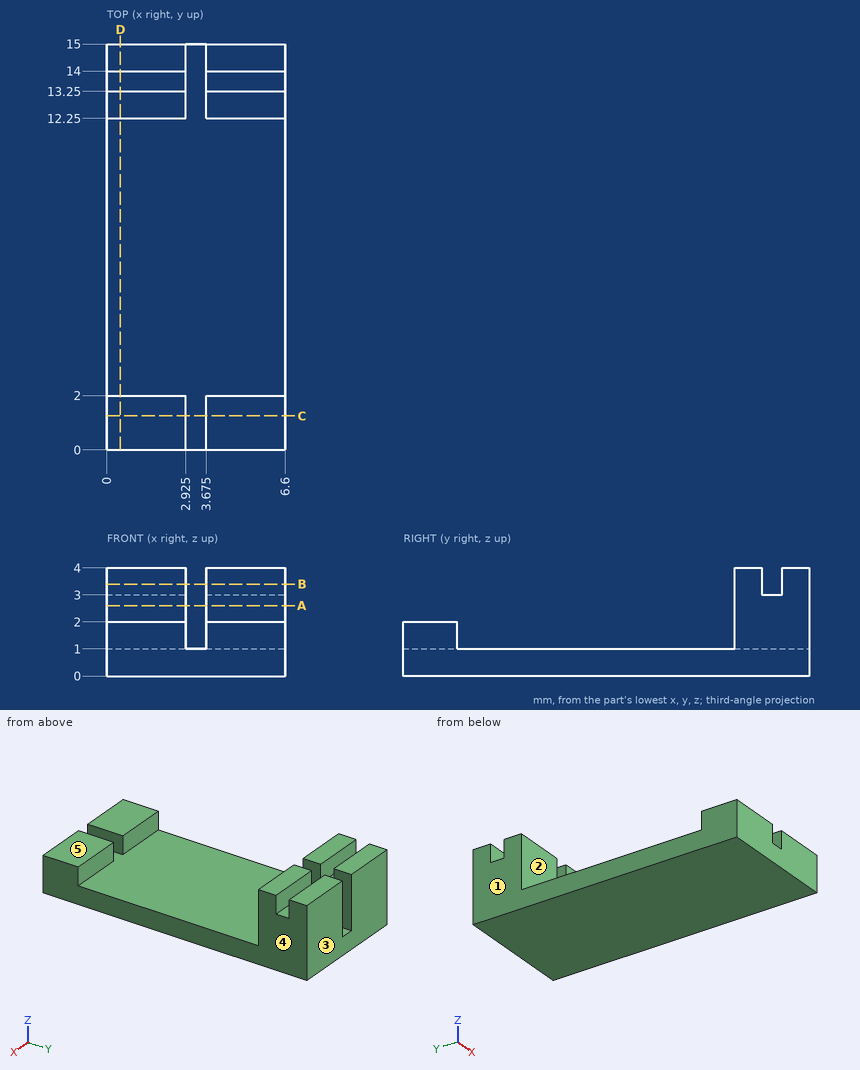
Study the drawing (mm; zero at the part's minimum x, y, z) and answer. A direction names the side the tool comes from. Round coordinates to 2 decimals unless told otherwise and drop trailing zeros. Write each loop counter-clockwise with the first axis right and the second up, starting at its lowest first coordinate (ties: lowest second). Pieces come first, ordered by that corner, then holes.
Q1. Find section D-D on x = 0.5. Determine the outline of the cut face in (y, z).
Values:
outline: (0, 0) - (15, 0) - (15, 4) - (14, 4) - (14, 3) - (13.25, 3) - (13.25, 4) - (12.25, 4) - (12.25, 1) - (2, 1) - (2, 2) - (0, 2) - close
Q2. Straight lines are drawn through the part: line 1 (Y direction, x = 5.25, z = 1.65); line 2 (X direction, y = 12.5, z = 3.45) (3 decimals); line 3 (Y direction, x = 3.75, z = 3.55). For each, find the intervals that lie inside material, in ascending order.
Values:
line 1: y = 0 to 2, 12.25 to 15
line 2: x = 0 to 2.925, 3.675 to 6.6
line 3: y = 12.25 to 13.25, 14 to 15
Q3. A tool of negligible diameter and unlimited length cuts with its end or side. For the marked faces 4 and 5, from which of +Z, -Z, +X, -X, +Y, -Y can it reach the whole face along a straight path? Write none if from no direction.
Values:
face 4: +Z, -Z, +X, +Y, -Y
face 5: +Z, +X, -X, -Y
Q4. Find section A-A on z = 2.6. Determine the outline of the cut face in (x, y) (3 decimals).
Values:
outline: (0, 12.25) - (2.925, 12.25) - (2.925, 15) - (0, 15) - close; (3.675, 12.25) - (6.6, 12.25) - (6.6, 15) - (3.675, 15) - close
Q5. Find section B-B on z = 3.4. Determine the outline of the cut face in (x, y) (3 decimals), and give its area (3 significant figures).
Values:
outline: (0, 12.25) - (2.925, 12.25) - (2.925, 13.25) - (0, 13.25) - close; (0, 14) - (2.925, 14) - (2.925, 15) - (0, 15) - close; (3.675, 12.25) - (6.6, 12.25) - (6.6, 13.25) - (3.675, 13.25) - close; (3.675, 14) - (6.6, 14) - (6.6, 15) - (3.675, 15) - close
area: 11.7 mm2
Q6. The mould has two halves that part along Y. Classify the marked faces 1, 2 and 3: released by +Y, released by -Y, zero draft, split by the parting line, or undercut.
Values:
face 1: zero draft
face 2: undercut
face 3: released by +Y
Q7. Flat-ended cylindrical pins translate along their axes: P1, Ø1.5, axis at x = 1, z = 3, coming from the -Y side; P2, Ø3.5, axis at x = 2.5, y = 6, coming from the +Z side; P3, Ø0.6, axis at x = 2, y = 1, coming from the +Z side. Find the tip coordinate at first contact, or state that the pin passes through.
Values:
P1: stops at y = 12.25
P2: stops at z = 1
P3: stops at z = 2
Q8. Find section C-C on y = 1.25. Determine the outline of the cut face in (x, z) (3 decimals).
Values:
outline: (0, 0) - (6.6, 0) - (6.6, 2) - (3.675, 2) - (3.675, 1) - (2.925, 1) - (2.925, 2) - (0, 2) - close
